from build123d import *

# Parameters (mm, degrees)
SKETCH1_R           = 2.2
BOSS_EXTRUDE1_DEPTH = 6.3


with BuildPart() as part:
    # Sketch1 → Boss-Extrude1 (new body)
    with BuildSketch(Plane.XY):
        with BuildLine():
            Line((-4, 0), (-4, 10))
            Line((-4, 10), (-1.65, 10))
            Line((-1.65, 10), (-1.65, 8))
            Line((-1.65, 8), (-2.75, 8))
            Line((-2.75, 8), (-2.75, 5.6))
            Line((-2.75, 5.6), (-1.65, 5.6))
            Line((-1.65, 5.6), (-1.65, 4))
            Line((-1.65, 4), (1.65, 4))
            Line((1.65, 4), (1.65, 5.6))
            Line((1.65, 5.6), (2.75, 5.6))
            Line((2.75, 5.6), (2.75, 8))
            Line((2.75, 8), (1.65, 8))
            Line((1.65, 8), (1.65, 10))
            Line((1.65, 10), (4, 10))
            Line((4, 10), (4, 0))
            ThreePointArc((4, 0), (0, -4), (-4, 0))
        make_face()
        Circle(SKETCH1_R, mode=Mode.SUBTRACT)
    extrude(amount=BOSS_EXTRUDE1_DEPTH)


solid = part.part
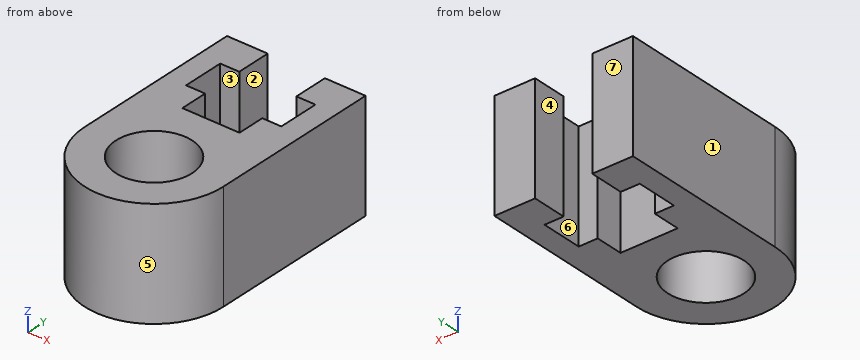
The model under review builds one solid part; all positions refer to its coordinate system, in mm. Face numbers are marked on the shaded views. A direction names the side the tool comes from. Give positions to 0.01 mm unless a question says otherwise; leave off trailing zeros. Order: outer loops, then holes, each group sorted by start corner. A loop starts at its lowest first (then second) coordinate and runs counter-clockwise, first axis right, second up. Notation, with made-up numbers: M 14.25,61 L 29.25,61 A35 cw 29.25,96 Z; hole C 87,79 d3. An arc over 180 degrees is marked long. Use one line per item in the form item = value. Start each with the question number.
Item 1: To check wall thickness, follow line 1 along X through (y, z) = (7.5, 4.25); line 2 along Y through (x, z) = (0, 5.5); line 3 along X through (y, z) = (5.25, 4.5). State the ranges of each line that lie inside material, in increasing order. Write a range as from..to.
Item 2: We need section D-D on x = 3.25. Give the boundary of the cut face in (y, z), plus the area to 3 significant figures.
Item 3: For the marked faces 1, 2 and 3, list the 3-axis set-ups (+Z, -Z, +X, -X, +Y, -Y) from which the entire face can be reached by the end or side of a thin tool; tool diameter is ignored.
Item 4: We need section C-C on z = 3. Give the boundary of the cut face in (x, y), plus the area to 3 significant figures.
Item 5: Insertion check: pin 1 Ø1 at (x, z) = (0, 4) entering from +Y; pin 2 Ø3 at (y, z) = (-2, 5) entering from +X; pin 3 Ø1.5 at (x, z) = (2.5, 2) entering from -Y. Each pin has a flat end and moves straight along its axis. Give the tip position at first contact, or say it passes through.
Item 6: We need section A-A on x = 0.75. Give the boundary of the cut face in (y, z).
Item 7: The part is to be moulded in two halves that separate along Y. For the marked faces 4, 5, 6 and 7, say which applies: pulls with the +Y half, pulls with the -Y half, needs draft (parallel to the pull), parting line crosses it, or undercut.
Item 8: We need section B-B on y = 7.75. Give the boundary of the cut face in (x, z), plus the area to 4 significant figures.
Completed:
q1.line_1 = -4..-2.75, 2.75..4
q1.line_2 = -4..-2.2, 2.2..4
q1.line_3 = -4..-1.65, 1.65..4
q2.outline = M -2.33,0 L 10,0 L 10,6.3 L -2.33,6.3 Z
q2.area = 77.7 mm²
q3.face_1 = +Z, -Z, -X, +Y, -Y
q3.face_2 = +Z, -Z, +Y
q3.face_3 = +Z, -Z
q4.outline = M -4,0 A4 ccw 4,0 L 4,10 L 1.65,10 L 1.65,8 L 2.75,8 L 2.75,5.6 L 1.65,5.6 L 1.65,4 L -1.65,4 L -1.65,5.6 L -2.75,5.6 L -2.75,8 L -1.65,8 L -1.65,10 L -4,10 Z; hole C 0,0 d4.4
q4.area = 64.8 mm²
q5.pin_1 = 4
q5.pin_2 = 3.97
q5.pin_3 = -3.6
q6.outline = M -3.93,0 L -2.07,0 L -2.07,6.3 L -3.93,6.3 Z; M 2.07,0 L 4,0 L 4,6.3 L 2.07,6.3 Z
q7.face_4 = needs draft
q7.face_5 = pulls with the -Y half
q7.face_6 = undercut
q7.face_7 = pulls with the +Y half
q8.outline = M -4,0 L -2.75,0 L -2.75,6.3 L -4,6.3 Z; M 2.75,0 L 4,0 L 4,6.3 L 2.75,6.3 Z
q8.area = 15.75 mm²
